The listing builds one solid part. Answer for the finished solid, in the listing's coordinates (mm). A direction names the side the tool comes from. Round coordinates to 2 decimals unless told otherwise and drop trailing zeros. Order: outer loops, then holes, each group sorted by start corner. A loop starts at its lowest first (then second) coordinate and runs counter-clockwise, first axis right, second up. Notation, with made-up numbers: (19, 62.5) - (73, 62.5) arc R20 ccw to (73, 97.5) - close; hole circle Ø4 at (67, -20.5). An arc over 180 degrees is marked (long way). One line per item, written item: value. Start each with the question number.
1. Section A-A, the plane y = -36 is taken. Give the vertices of the cut face in (x, z).
2. A flat-ended cylindrical pin translates along its axis: P1, Ø12, axis at x = -5.5, y = 15, coming from the -Z side. Find the tip coordinate at first contact, or state that the pin passes through.
3. Section C-C, the plane z = 0 is taken. Give the vertices of the cut face in (x, y), then the cut area to 3 significant figures.
4. Section B-B, the plane x = 0 is taken. Give the vertices of the cut face in (y, z).
5. For a pull along X with two mould halves and no side action, classify faces 1 (the flat face through (9.5, -7, 0)), 2 (the flat face through (12.5, -2, 0)), 3 (the cylindrical face through (-7.4, -39.1, 0)), 4 (the flat face through (-10, 47.5, 0)) as released by +X, released by -X, zero draft, split by the parting line, or undercut.
6. Straight lines are drawn through the part: line 1 (X direction, y = -6.5, z = 1.15); line 2 (Y direction, x = 0, z = -0.7); line 3 (Y direction, x = 8, z = -1.4). For each, find the intervals that lie inside material, in ascending order.
7. A tool of negligible diameter and unlimited length cuts with its end or side. For faces 5 (the flat face through (5.3, -7, 0)), 6 (the flat face through (0, 1, -2.5)), from which of +Z, -Z, +X, -X, +Y, -Y can it reach the whole face along a straight path? Write none if from no direction.
8. Section D-D, the plane y = 37 is taken. Give the vertices of the cut face in (x, z), then the cut area to 3 significant figures.
from build123d import *

# Parameters (mm, degrees)
SKETCH1_R           = 9.25
BOSS_EXTRUDE1_DEPTH = 2.5


with BuildPart() as part:
    # Sketch1 → Boss-Extrude1 (new, symmetric)
    with BuildSketch(Plane.XY):
        Polygon((-7.5, 50), (7.5, 50), (12.5, 45), (12.5, -50), (-12.5, -50), (-12.5, 45), align=None)
        with Locations((0, 37)):
            Circle(SKETCH1_R, mode=Mode.SUBTRACT)
        with BuildLine():
            Line((9.5, 23), (9.5, -37))
            ThreePointArc((9.5, -37), (7.4, -39.1), (5.3, -37))
            Line((5.3, -37), (5.3, 23))
            ThreePointArc((5.3, 23), (7.4, 25.1), (9.5, 23))
        make_face(mode=Mode.SUBTRACT)
        with BuildLine():
            Line((-9.5, 23), (-9.5, -37))
            ThreePointArc((-9.5, -37), (-7.4, -39.1), (-5.3, -37))
            Line((-5.3, -37), (-5.3, 23))
            ThreePointArc((-5.3, 23), (-7.4, 25.1), (-9.5, 23))
        make_face(mode=Mode.SUBTRACT)
    extrude(amount=BOSS_EXTRUDE1_DEPTH, both=True)


solid = part.part
Answer list:
1. outline: (-12.5, -2.5) - (-9.5, -2.5) - (-9.5, 2.5) - (-12.5, 2.5) - close; (-5.3, -2.5) - (5.3, -2.5) - (5.3, 2.5) - (-5.3, 2.5) - close; (9.5, -2.5) - (12.5, -2.5) - (12.5, 2.5) - (9.5, 2.5) - close
2. P1: stops at z = -2.5
3. outline: (-12.5, -50) - (12.5, -50) - (12.5, 45) - (7.5, 50) - (-7.5, 50) - (-12.5, 45) - close; hole (-9.5, -37) arc R2.1 ccw to (-5.3, -37) - (-5.3, 23) arc R2.1 ccw to (-9.5, 23) - close; hole circle Ø18.5 at (0, 37); hole (5.3, -37) arc R2.1 ccw to (9.5, -37) - (9.5, 23) arc R2.1 ccw to (5.3, 23) - close
3. area: 1,670 mm²
4. outline: (-50, -2.5) - (27.75, -2.5) - (27.75, 2.5) - (-50, 2.5) - close; (46.25, -2.5) - (50, -2.5) - (50, 2.5) - (46.25, 2.5) - close
5. face 1: undercut
5. face 2: released by +X
5. face 3: undercut
5. face 4: released by -X
6. line 1: x = -12.5 to -9.5, -5.3 to 5.3, 9.5 to 12.5
6. line 2: y = -50 to 27.75, 46.25 to 50
6. line 3: y = -50 to -39.01, 25.01 to 32.36, 41.64 to 49.5
7. face 5: +Z, -Z
7. face 6: -Z, +X, -X, +Y, -Y
8. outline: (-12.5, -2.5) - (-9.25, -2.5) - (-9.25, 2.5) - (-12.5, 2.5) - close; (9.25, -2.5) - (12.5, -2.5) - (12.5, 2.5) - (9.25, 2.5) - close
8. area: 32.5 mm²
